Source: CAD feature listing. Evaluate the final solid. Frame: model axes, mm. A direction names the side the tool comes from. Round coordinates to 2 decimals unless told otherwise and drop trailing zeros. Loops run counter-clockwise (first coordinate to the right, second up) from the corner with the lowest first, then second, coordinate; pieces in that order, holes last.
Item 1: Pull-direction query (X, two-part tool) for faces 1 (the flat face through (-4, -6, 16)), 2 (the cylindrical face through (11.19, -0.06, 62.72)), 3 (the flat face through (0, -10.7, 33)); classes: released by +X, released by -X, zero draft, split by the parting line, or undercut.
Item 2: Section query D-D on x = -2. Return loops of the section in (y, z), then the cut area to 3 significant figures.
Item 3: Section query C-C on x = 6.5. Return loops of the section in (y, z), then the cut area to 3 significant figures.
Item 4: First-contact query: P1, Ø5, axis at x = -12.5, y = 37, coming from the -Z side; P2, Ø2, axis at x = 9, y = -12.5, coming from the +Z side; P3, Ø1.8, axis at x = 1, z = 32.5, coming from the -Y side; P4, Ø1.5, axis at y = 13, z = 49, coming from the -X side. Flat tips, straight axial feed; report the tip coordinate or a pass-through.
Item 5: Section query A-A on y = 45. Return loops of the section in (x, z).
Item 6: Section query B-B on z = 18. Return loops of the section in (x, y), then the cut area to 3 significant figures.
Item 7: Ray query, L1, parallel to X at y = 37, z = 28; L2, parallel to Y at x = 8.75, z = 15.7; L3, parallel to X at y = -12, z = 25. Return the intervals inside material, ascending.
Item 8: Access query for faces 4 (the flat face through (-14, 15.7, 16)), 5 (the flat face through (-9.5, 41, 28)), 6 (the flat face through (-13, 44, 22)). Directions: +Z, -Z, +X, -X, +Y, -Y. A direction counts if a zero-diameter tool reaches every point of the face in a straight line with its end or side. Return the directions, or none.
```python
from build123d import *

# Parameters (mm, degrees)
SKETCH4_W            = 31.4
SKETCH4_H            = 31.4
SKETCH4_W_2          = 25.4
SKETCH4_H_2          = 25.4
BOSS_EXTRUDE3_DEPTH  = 30
SKETCH5_W            = 31.4
SKETCH5_H            = 31.4
BOSS_EXTRUDE4_DEPTH  = 5
SKETCH6_W            = 31.4
SKETCH6_H            = 8
BOSS_EXTRUDE5_DEPTH  = 5
BOSS_EXTRUDE6_DEPTH  = 8
SKETCH8_R            = 4
BOSS_EXTRUDE7_DEPTH  = 8
SKETCH9_W            = 31.4
SKETCH9_H            = 10
BOSS_EXTRUDE8_DEPTH  = 5
SKETCH10_W           = 31.4
SKETCH10_H           = 10
BOSS_EXTRUDE9_DEPTH  = 13
SKETCH11_W           = 6.2
SKETCH11_H           = 10
BOSS_EXTRUDE10_DEPTH = 40
BOSS_EXTRUDE11_DEPTH = 3
SKETCH13_W           = 31.4
SKETCH13_H           = 31.4
CUT_EXTRUDE1_DEPTH   = 31.4
SKETCH15_W           = 31.4
SKETCH15_H           = 13
BOSS_EXTRUDE12_DEPTH = 12
SKETCH17_W           = 8
SKETCH17_H           = 31.4
BOSS_EXTRUDE13_DEPTH = 10
SKETCH18_R           = 4
BOSS_EXTRUDE14_DEPTH = 8
SKETCH19_W           = 3.6
SKETCH19_H           = 5
CUT_EXTRUDE2_DEPTH   = 31.4
SKETCH20_W           = 8
SKETCH20_H           = 1
CUT_EXTRUDE3_DEPTH   = 26.4


with BuildPart() as part:
    # Sketch4 → Boss-Extrude3 (new body)
    with BuildSketch(Plane.XY):
        Rectangle(SKETCH4_W, SKETCH4_H)
        Rectangle(SKETCH4_W_2, SKETCH4_H_2, mode=Mode.SUBTRACT)
    extrude(amount=BOSS_EXTRUDE3_DEPTH)

    # Sketch5 → Boss-Extrude4 (add)
    with BuildSketch(Plane.XY.offset(30)):
        Rectangle(SKETCH5_W, SKETCH5_H)
    extrude(amount=BOSS_EXTRUDE4_DEPTH)

    # Sketch6 → Boss-Extrude5 (add)
    with BuildSketch(Plane.XY.offset(35)):
        Rectangle(SKETCH6_W, SKETCH6_H)
    extrude(amount=BOSS_EXTRUDE5_DEPTH)

    # Sketch7 → Boss-Extrude6 (add)
    with BuildSketch(Plane.XZ.offset(4)):
        with BuildLine():
            Line((-15.7, 40), (-15.7, 52))
            ThreePointArc((-15.7, 52), (-11.306601718, 62.606601718), (-0.7, 67))
            Line((-0.7, 67), (0.7, 67))
            ThreePointArc((0.7, 67), (11.306601718, 62.606601718), (15.7, 52))
            Line((15.7, 52), (15.7, 40))
            Line((15.7, 40), (-15.7, 40))
        make_face()
    extrude(amount=-BOSS_EXTRUDE6_DEPTH)

    # Sketch8 → Boss-Extrude7 (add)
    with BuildSketch(Plane.XZ.offset(4)):
        with Locations(Location((0, 52, 0), (0, 0, 180))):
            Circle(SKETCH8_R)
    boss_extrude7 = extrude(amount=BOSS_EXTRUDE7_DEPTH)

    # Mirror1: Boss-Extrude7 across plane
    add(boss_extrude7.mirror(Plane.ZX))

    # Sketch9 → Boss-Extrude8 (add)
    with BuildSketch(Plane(origin=(0, 15.7, 0), x_dir=(1, 0, 0), z_dir=(0, 1, 0))):
        with Locations((0, -27)):
            Rectangle(SKETCH9_W, SKETCH9_H)
    extrude(amount=BOSS_EXTRUDE8_DEPTH)

    # Sketch10 → Boss-Extrude9 (add)
    with BuildSketch(Plane(origin=(0, 15.7, 0), x_dir=(1, 0, 0), z_dir=(0, 1, 0))):
        with Locations((0, -17)):
            Rectangle(SKETCH10_W, SKETCH10_H)
    extrude(amount=BOSS_EXTRUDE9_DEPTH)

    # Sketch11 → Boss-Extrude10 (add)
    with BuildSketch(Plane(origin=(0, 20.7, 0), x_dir=(1, 0, 0), z_dir=(0, 1, 0))):
        with Locations((-12.6, -27)):
            Rectangle(SKETCH11_W, SKETCH11_H)
        with Locations((12.6, -27)):
            Rectangle(SKETCH11_W, SKETCH11_H)
    extrude(amount=BOSS_EXTRUDE10_DEPTH)

    # Sketch12 → Boss-Extrude11 (add)
    with BuildSketch(Plane.XY.offset(32)):
        Polygon((-15.7, 60.7), (-9.5, 60.7), (-9.5, 20.7), (9.5, 20.7), (9.5, 60.7), (15.7, 60.7), (15.7, 15.7), (-15.7, 15.7), align=None)
    extrude(amount=BOSS_EXTRUDE11_DEPTH)

    # Sketch13 → Cut-Extrude1 (cut)
    with BuildSketch(Plane.ZY.offset(15.7)):
        with Locations((15.7, 0)):
            Rectangle(SKETCH13_W, SKETCH13_H)
    extrude(amount=-CUT_EXTRUDE1_DEPTH, mode=Mode.SUBTRACT)

    # Sketch15 → Boss-Extrude12 (add)
    with BuildSketch(Plane(origin=(0, 0, 12), x_dir=(-1, 0, 0), z_dir=(0, 0, -1))):
        with Locations((0, 22.2)):
            Rectangle(SKETCH15_W, SKETCH15_H)
    extrude(amount=BOSS_EXTRUDE12_DEPTH)

    # Sketch17 → Boss-Extrude13 (add)
    with BuildSketch(Plane.XZ.offset(-15.7)):
        with Locations((-8, 15.7)):
            Rectangle(SKETCH17_W, SKETCH17_H)
    boss_extrude13 = extrude(amount=BOSS_EXTRUDE13_DEPTH)

    # Sketch18 → Boss-Extrude14 (add)
    with BuildSketch(Plane.ZY.offset(12)):
        with BuildLine():
            Line((31.4, 5.7), (0, 5.7))
            Line((0, 5.7), (0, -13.3))
            ThreePointArc((0, -13.3), (4.393398282, -23.906601718), (15, -28.3))
            Line((15, -28.3), (16.4, -28.3))
            ThreePointArc((16.4, -28.3), (27.006601718, -23.906601718), (31.4, -13.3))
            Line((31.4, -13.3), (31.4, 5.7))
        make_face()
        with Locations((15.7, -13.3)):
            Circle(SKETCH18_R, mode=Mode.SUBTRACT)
    boss_extrude14 = extrude(amount=-BOSS_EXTRUDE14_DEPTH)

    # Mirror3: Boss-Extrude13, Boss-Extrude14 across plane
    add(boss_extrude13.mirror(Plane(origin=(0, 0, 0), x_dir=(0, 0, 1), z_dir=(1, 0, 0))))
    add(boss_extrude14.mirror(Plane(origin=(0, 0, 0), x_dir=(0, 0, 1), z_dir=(1, 0, 0))))

    # Sketch19 → Cut-Extrude2 (cut)
    with BuildSketch(Plane(origin=(15.7, 0, 0), x_dir=(0, 0, -1), z_dir=(1, 0, 0))):
        with Locations((-33.2, -13.2)):
            Rectangle(SKETCH19_W, SKETCH19_H)
    extrude(amount=-CUT_EXTRUDE2_DEPTH, mode=Mode.SUBTRACT)

    # Sketch20 → Cut-Extrude3 (cut)
    with BuildSketch(Plane.XZ.offset(10.7)):
        with Locations((0, 31.9)):
            Rectangle(SKETCH20_W, SKETCH20_H)
    extrude(amount=-CUT_EXTRUDE3_DEPTH, mode=Mode.SUBTRACT)


solid = part.part
```
Data:
1. face 1: undercut
1. face 2: released by +X
1. face 3: zero draft
2. outline: (-12, 48.54) - (-4, 48.54) - (-4, 35) - (-10.7, 35) - (-10.7, 32.4) - (15.7, 32.4) - (15.7, 0) - (28.7, 0) - (28.7, 22) - (20.7, 22) - (20.7, 35) - (4, 35) - (4, 48.54) - (12, 48.54) - (12, 55.46) - (4, 55.46) - (4, 66.94) - (-4, 66.94) - (-4, 55.46) - (-12, 55.46) - close
2. area: 786 mm2
3. outline: (-28.3, 15) arc R15 ccw to (-13.3, 0) - (28.7, 0) - (28.7, 22) - (20.7, 22) - (20.7, 35) - (4, 35) - (4, 65.83) - (-4, 65.83) - (-4, 35) - (-10.7, 35) - (-10.7, 31.4) - (-13.3, 31.4) arc R15 ccw to (-28.3, 16.4) - close; hole circle Ø8 at (-13.3, 15.7)
3. area: 1,930 mm2
4. P1: stops at z = 22
4. P2: stops at z = 31.4
4. P3: stops at y = -10.7
4. P4: passes through
5. outline: (-15.7, 22) - (-9.5, 22) - (-9.5, 35) - (-15.7, 35) - close; (9.5, 22) - (15.7, 22) - (15.7, 35) - (9.5, 35) - close
6. outline: (-15.7, 15.7) - (-12, 15.7) - (-12, -10.03) - (-4, -10.03) - (-4, 15.7) - (4, 15.7) - (4, -10.03) - (12, -10.03) - (12, 15.7) - (15.7, 15.7) - (15.7, 28.7) - (-15.7, 28.7) - close; (-12, -28.21) - (-4, -28.21) - (-4, -16.57) - (-12, -16.57) - close; (4, -28.21) - (12, -28.21) - (12, -16.57) - (4, -16.57) - close
6. area: 1,010 mm2
7. L1: x = -15.7 to -9.5, 9.5 to 15.7
7. L2: y = -28.3 to -17.3, -9.3 to 28.7
7. L3: x = -12 to -4, 4 to 12
8. face 4: -Z, -X, -Y
8. face 5: +Z, +Y
8. face 6: -Z, +X, -X, +Y
